For this review, take the finished solid that the model builds, in its own axes (mm). A direction names the side the tool comes from. Give positions to 0.01 mm unless a question says otherwise; leave off trailing zeros. Order: outer loops, then holes, each group sorted by start corner. A loop starts at its lowest first (then second) coordinate and runs counter-clockwise, first axis right, second up.
from build123d import *

# Parameters (mm, degrees)
SKETCH_W         = 150
SKETCH_H         = 65
SKETCH_W_2       = 101
SKETCH_H_2       = 51
PAD_DEPTH        = 1.5
SKETCH001_W      = 150
SKETCH001_H      = 65
PAD001_DEPTH     = 8.5
HOLE_D           = 5
HOLE_DEPTH       = 25
HOLE_CSINK_D     = 10
HOLE_CSINK_ANGLE = 90


with BuildPart() as part:
    # Sketch → Pad (new body)
    with BuildSketch(Plane.XY):
        Rectangle(SKETCH_W, SKETCH_H)
        Rectangle(SKETCH_W_2, SKETCH_H_2, mode=Mode.SUBTRACT)
    extrude(amount=PAD_DEPTH)

    # Sketch001 (on Face10 of Pad) → Pad001 (join)
    with BuildSketch(Plane.XY.offset(1.5)):
        Rectangle(SKETCH001_W, SKETCH001_H)
    extrude(amount=PAD001_DEPTH)

    # Hole
    with Locations(Plane(origin=(0, 0, 0), x_dir=(1, 0, 0), z_dir=(0, 0, -1))):
        with Locations((-65, 22.5), (-65, -22.5), (65, 22.5), (65, -22.5)):
            CounterSinkHole(HOLE_D / 2, HOLE_CSINK_D / 2, depth=HOLE_DEPTH, counter_sink_angle=HOLE_CSINK_ANGLE)


solid = part.part
1) We need section C-C on x = -9. Give the boundary of the cut face in (y, z), then the cut area to 4 significant figures.
Answer sheet:
outline: (-32.5, 0) - (-25.5, 0) - (-25.5, 1.5) - (25.5, 1.5) - (25.5, 0) - (32.5, 0) - (32.5, 10) - (-32.5, 10) - close
area: 573.5 mm2
2) Draft analysis for pull direction X (two halves, no side actions). For faces 1 (the face through (-75, 0, 5)), 2 (the face through (-62.38, -22.62, 2.38)), 3 (the face through (75, 0, 5)), state which applies: +X half, -X half, draft (parallel to the pull), parting line (faces both ways), or undercut.
Answer sheet:
face 1: -X half
face 2: undercut
face 3: +X half
3) We need section D-D on y = -11. Give the boundary of the cut face in (x, z), then the cut area to 3 significant figures.
Answer sheet:
outline: (-75, 0) - (-50.5, 0) - (-50.5, 1.5) - (50.5, 1.5) - (50.5, 0) - (75, 0) - (75, 10) - (-75, 10) - close
area: 1,350 mm2
4) Tool access review of faces 4 (the face through (63.66, 20.39, 6.3)), 5 (the face through (-1, 0, 1.5)): name each direction out of +Z, -Z, +X, -X, +Y, -Y from which nothing blocks a thin tool from reaching the whole face with its end or side.
Answer sheet:
face 4: +Z, -Z
face 5: -Z
5) To check wall thickness, follow line 1 (Y direction, x = -65, z = 4.75); line 2 (X direction, y = -22.5, z = 5); line 3 (Y direction, x = -48, z = 1). State the ranges of each line that lie inside material, in increasing order.
Answer sheet:
line 1: y = -32.5 to -25, -20 to 20, 25 to 32.5
line 2: x = -75 to -67.5, -62.5 to 62.5, 67.5 to 75
line 3: y = -32.5 to -25.5, 25.5 to 32.5
6) We need section B-B on x = 65. Give the boundary of the cut face in (y, z), then the cut area to 4 significant figures.
Answer sheet:
outline: (-32.5, 0) - (-27.5, 0) - (-25, 2.5) - (-25, 10) - (-32.5, 10) - close; (-20, 2.5) - (-17.5, 0) - (17.5, 0) - (20, 2.5) - (20, 10) - (-20, 10) - close; (25, 2.5) - (27.5, 0) - (32.5, 0) - (32.5, 10) - (25, 10) - close
area: 537.5 mm2
7) We need section A-A on y = 22.5. Give the boundary of the cut face in (x, z), then the cut area to 3 significant figures.
Answer sheet:
outline: (-75, 0) - (-70, 0) - (-67.5, 2.5) - (-67.5, 10) - (-75, 10) - close; (-62.5, 2.5) - (-60, 0) - (-50.5, 0) - (-50.5, 1.5) - (50.5, 1.5) - (50.5, 0) - (60, 0) - (62.5, 2.5) - (62.5, 10) - (-62.5, 10) - close; (67.5, 2.5) - (70, 0) - (75, 0) - (75, 10) - (67.5, 10) - close
area: 1,240 mm2
8) Clearance check with flat-ended pins moving along their axes: pin 1 (3 mm diameter, centred on x = -30.5, y = -16, fed in from -Z); pin 2 (6 mm diameter, centred on x = 65, y = -22.5, fed in from -Z); pin 3 (6.5 mm diameter, centred on x = 65, y = 22.5, fed in from -Z); pin 4 (3 mm diameter, centred on x = -65, y = 22.5, fed in from +Z). State where each tip first meets the part, or that it passes through.
Answer sheet:
pin 1: stops at z = 1.5
pin 2: stops at z = 2
pin 3: stops at z = 1.75
pin 4: passes through
